Read the model definition and answer for the solid it produces. Units are mm, in the model's axes. A direction names the side the tool comes from. Coordinates: 2 decimals unless noted, no trailing zeros. Write each loop counter-clockwise with the first axis right and the second up, starting at its lowest first coordinate (ties: lowest second). Pieces come first, ordered by that corner, then holes. Notation, with made-up numbers: (76.25, 15) - (101.25, 15) arc R22 ccw to (101.25, 44) - close; hole circle Ø10 at (-27.75, 81). An arc over 180 degrees is marked (long way). Use a Markdown table: item, result.
from build123d import *

# Parameters (mm, degrees)
MODEL_R            = 6.45
MODEL_W            = 1.905
MODEL_H            = 2.794
BOSS_EXTRU_1_DEPTH = 1.6


with BuildPart() as part:
    # Model → Boss.-Extru.1 (new body)
    with BuildSketch(Plane.XY):
        Circle(MODEL_R)
        with Locations((-2.54, -3)):
            Rectangle(MODEL_W, MODEL_H, mode=Mode.SUBTRACT)
        with BuildLine():
            Line((0.9525, -2.5555), (0.9525, -3.4445))
            ThreePointArc((0.9525, -3.4445), (0, -4.397), (-0.9525, -3.4445))
            Line((-0.9525, -3.4445), (-0.9525, -2.5555))
            ThreePointArc((-0.9525, -2.5555), (0, -1.603), (0.9525, -2.5555))
        make_face(mode=Mode.SUBTRACT)
        with BuildLine():
            Line((3.4925, -2.5555), (3.4925, -3.4445))
            ThreePointArc((3.4925, -3.4445), (2.54, -4.397), (1.5875, -3.4445))
            Line((1.5875, -3.4445), (1.5875, -2.5555))
            ThreePointArc((1.5875, -2.5555), (2.54, -1.603), (3.4925, -2.5555))
        make_face(mode=Mode.SUBTRACT)
    extrude(amount=BOSS_EXTRU_1_DEPTH)


solid = part.part
(1) Straight lines are drawn through the part: L1, parallel to Y at x = 2.75, z = 0.3; L2, parallel to Y at x = -2.5, z = 0.45; L3, parallel to Y at x = -3.75, z = 1.35. For each, find the intervals that lie inside material, in ascending order.
Report:
| item | result |
|---|---|
| L1 | y = -5.83 to -4.37, -1.63 to 5.83 |
| L2 | y = -5.95 to -4.4, -1.6 to 5.95 |
| L3 | y = -5.25 to 5.25 |
(2) A cutting plane is placed at D-D, the plane y = 2.75. Write down the section's boundary in (x, z), and give its area (3 significant figures).
Report:
| item | result |
|---|---|
| outline | (-5.83, 0) - (5.83, 0) - (5.83, 1.6) - (-5.83, 1.6) - close |
| area | 18.7 mm² |
(3) A cutting plane is placed at A-A, the plane x = 0. Write down the section's boundary in (y, z).
Report:
| item | result |
|---|---|
| outline | (-6.45, 0) - (-4.4, 0) - (-4.4, 1.6) - (-6.45, 1.6) - close; (-1.6, 0) - (6.45, 0) - (6.45, 1.6) - (-1.6, 1.6) - close |
(4) A cutting plane is placed at C-C, the plane x = -1.75. Write down the section's boundary in (y, z), and give its area (3 significant figures).
Report:
| item | result |
|---|---|
| outline | (-6.21, 0) - (-4.4, 0) - (-4.4, 1.6) - (-6.21, 1.6) - close; (-1.6, 0) - (6.21, 0) - (6.21, 1.6) - (-1.6, 1.6) - close |
| area | 15.4 mm² |
(5) A cutting plane is placed at B-B, the plane z = 0.95. Count the separate pieces of the cut face and the enclosed holes in it, and give its area (3 significant figures).
Report:
| item | result |
|---|---|
| separate pieces | 1 |
| enclosed holes | 3 |
| area | 116 mm² |
(6) For faces 1 (the flat face through (-3.492, -3, 1)), 2 (the flat face through (0, 0, 1.6)), determine the directions among +Z, -Z, +X, -X, +Y, -Y from which every point of the face is accessible in a straight line to the end or side of a thin tool.
Report:
| item | result |
|---|---|
| face 1 | +Z, -Z |
| face 2 | +Z, +X, -X, +Y, -Y |
(7) Each of these flat-tipped pins is pushed along its axis until it touches: P1, Ø0.8, axis at y = -3.5, z = 1, coming from the +X side; P2, Ø0.7, axis at y = -3, z = 0.5, coming from the +X side; P3, Ø0.5, axis at x = -3, z = 0.5, coming from the -Y side. Where does it stop, or does it pass through?
Report:
| item | result |
|---|---|
| P1 | stops at x = 5.66 |
| P2 | stops at x = 5.88 |
| P3 | stops at y = -5.83 |
(8) The mould has two halves that part along Y. Classify faces 3 (the flat face through (0, 0, 0)), 4 (the flat face through (0.952, -3, 1)), 5 (the cylindrical face through (-1.398, -6.297, 0.789)): pulls with the +Y half, pulls with the -Y half, needs draft (parallel to the pull), parting line crosses it, or undercut.
Report:
| item | result |
|---|---|
| face 3 | needs draft |
| face 4 | undercut |
| face 5 | parting line crosses it |
